Source: CAD feature listing. Evaluate the final solid. Frame: model axes, mm. A direction names the side the tool comes from. Coordinates: 2 decimals unless noted, no trailing zeros. Order: outer loops, then holes, each group sorted by start corner. A loop starts at its lowest first (then second) coordinate and runs counter-clockwise, first axis right, second up.
```python
from build123d import *

# Parameters (mm, degrees)
F1_DEPTH = 20


with BuildPart() as f1:
    # F0 (on Front) → F1 (new body)
    with BuildSketch(Plane.XZ):
        with BuildLine():
            Line((-20, 0), (0, 0))
            Line((0, 0), (0, 191))
            ThreePointArc((0, 191), (-2.828427, 192.171573), (-4, 195))
            Line((-4, 195), (-6, 195))
            ThreePointArc((-6, 195), (-8.828427, 193.828427), (-10, 191))
            Line((-10, 191), (-10, 6))
            ThreePointArc((-10, 6), (-10.87868, 3.87868), (-13, 3))
            Line((-13, 3), (-19, 3))
            ThreePointArc((-19, 3), (-19.707107, 2.707107), (-20, 2))
            Line((-20, 2), (-20, 0))
        make_face()
    extrude(amount=F1_DEPTH)

    # F2: F1 across face


with BuildPart() as f1_1:
    add(f1.part)
    add(f1.part.mirror(Plane(origin=(0, -10, 95.5), x_dir=(0, 1, 0), z_dir=(1, 0, 0))))


solid = f1_1.part
```
1. Section query C-C on x = 15. Return loops of the section in (y, z).
Findings:
outline: (-20, 0) - (0, 0) - (0, 3) - (-20, 3) - close
2. Ray query, line 1 (X direction, y = -18, z = 14); line 2 (Z direction, x = -14.5, y = -15.5); line 3 (Z direction, x = 6.5, y = -3.25). Return the intervals inside material, ascending.
Findings:
line 1: x = -10 to 10
line 2: z = 0 to 3
line 3: z = 0 to 194.97
3. Section query A-A on y = -2.5. Return loops of the section in (x, z).
Findings:
outline: (-20, 0) - (20, 0) - (20, 2) arc R1 ccw to (19, 3) - (13, 3) arc R3 cw to (10, 6) - (10, 191) arc R4 ccw to (6, 195) - (4, 195) arc R4 cw to (-4, 195) - (-6, 195) arc R4 ccw to (-10, 191) - (-10, 6) arc R3 cw to (-13, 3) - (-19, 3) arc R1 ccw to (-20, 2) - close
4. Pin query (flat end, axial travel): P1, Ø6, axis at y = -8, z = 141, coming from the -X side; P2, Ø1.8, axis at x = 14.5, y = -9, coming from the +Z side; P3, Ø10, axis at y = -12, z = 115.5, coming from the +X side. Return the tip coordinate at first contact, or that it passes through.
Findings:
P1: stops at x = -10
P2: stops at z = 3
P3: stops at x = 10
5. Section query B-B on z = 102.5. Return loops of the section in (x, y).
Findings:
outline: (-10, -20) - (10, -20) - (10, 0) - (-10, 0) - close
6. Access query for faces 1 (the face through (10, -10, 100)), 2 (the face through (-16, -10, 3)), 3 (the face through (0, 0, 99)). Directions: +Z, -Z, +X, -X, +Y, -Y. A direction counts if a zero-diameter tool reaches every point of the face in a straight line with its end or side. Return the directions, or none.
Findings:
face 1: +Z, +X, +Y, -Y
face 2: +Z, -X, +Y, -Y
face 3: +Z, -Z, +X, -X, +Y
